Can you work these out from the model? Positions are in its coordinate system, mm. A direction names the side the tool comes from. Give positions to 0.01 mm unless a question says otherwise; leave off trailing zeros. Loops run counter-clockwise (first coordinate to the right, second up) from the corner with the lowest first, then second, coordinate; pieces in that order, holes last. Notation, with made-up numbers: M 81.5,65.25 L 119.5,65.25 A33 cw 119.5,95.25 Z; hole C 50,16 d11. An arc over 180 degrees is marked long. Use CSV: the item, a comma, the result in double quotes.
Autodesk Fusion 360 part; units mm, degrees
sketch "Sketch1" plane through (0, 0, 0) normal (0, 1, 0) x (1, 0, 0)
  line L0 (-6.9154, 10.127) -> (7.6855, 10.127)
  line L1 (7.6855, 10.127) -> (7.6855, -8.5945)
  line L2 (7.6855, -8.5945) -> (-6.9154, -8.5945)
  line L3 (-6.9154, -8.5945) -> (-6.9154, 10.127)
extrude "Extrude1" add sketch "Sketch1" along normal blind 6
sketch "Sketch2" plane through (0, 0, 0) normal (0, -1, 0) x (1, 0, 0)
  line L0 (7.6855, 8.5945) -> (-6.9154, 8.5945)
  line L1 (-6.9154, 8.5945) -> (-6.9154, -10.127)
  line L2 (-6.9154, -10.127) -> (7.6855, -10.127)
  line L3 (7.6855, -10.127) -> (7.6855, 8.5945)
  line L4 (-6.9154, 8.5945) -> (-4.4154, 8.5945)
  line L5 (7.6855, 8.5945) -> (5.1855, 8.5945)
  line L6 (-4.4154, 8.5945) -> (-4.4154, 7.6945)
  line L7 (5.1855, 8.5945) -> (5.1855, 7.6945)
  line L8 (5.1855, 7.6945) -> (5.1855, 3.6245)
  line L9 (-4.4154, 7.6945) -> (5.1855, 7.6945)
  line L10 (5.1855, 7.6945) -> (5.1855, 3.6245)
  line L11 (5.1855, 3.6245) -> (-4.4154, 3.6245)
  line L12 (-4.4154, 3.6245) -> (-4.4154, 7.6945)
  dimension "d3" = 2.5
  dimension "d4" = 2.5
  dimension "d5" = 0.9
  dimension "d6" = 0.9
  dimension "d7" = 4.07
extrude "Extrude2" cut sketch "Sketch2" against normal blind 4.5 contours L8 L9 L10 L11 L12
sketch "Sketch3" plane through (-6.9154, 0, 0) normal (-1, 0, 0) x (0, 0, 1)
  line L0 (-10.127, 0) -> (8.5945, 0)
  line L1 (8.5945, 0) -> (8.5945, 6)
  line L2 (8.5945, 6) -> (-10.127, 6)
  line L3 (-10.127, 6) -> (-10.127, 0)
  line L4 (8.5945, 0) -> (3.6345, 0)
  line L5 (8.5945, 0) -> (7.6945, 0)
  line L6 (7.6945, 0) -> (7.6945, 4.5)
  line L7 (3.6345, 0) -> (3.6245, 4.5)
  dimension "d10" = 4.96
  dimension "d11" = 0.9
  dimension "d12" = 4.5
sketch "Sketch4" plane through (0, 6, 0) normal (0, 1, 0) x (-1, 0, 0)
  line L0 (6.9154, 8.5945) -> (-7.6855, 8.5945)
  line L1 (-7.6855, 8.5945) -> (-7.6855, -10.127)
  line L2 (-7.6855, -10.127) -> (6.9154, -10.127)
  line L3 (6.9154, -10.127) -> (6.9154, 8.5945)
  line L4 (6.9154, 8.5945) -> (4.9154, 8.5945)
  line L5 (-7.6855, 8.5945) -> (-5.6855, 8.5945)
  line L6 (6.9154, -10.127) -> (4.9154, -10.127)
  line L7 (-7.6855, -10.127) -> (-5.6855, -10.127)
  line L8 (4.9154, -10.127) -> (-5.6855, -10.127)
  line L9 (-5.6855, -10.127) -> (-5.6855, 8.5945)
  line L10 (-5.6855, 8.5945) -> (4.9154, 8.5945)
  line L11 (4.9154, 8.5945) -> (4.9154, -10.127)
  dimension "d13" = 2
  dimension "d14" = 2
  dimension "d15" = 2
  dimension "d16" = 2
extrude "Extrude3" cut sketch "Sketch4" against normal up to surface (1.5 mm away) contours L0 L2 L8 L9 L10 L11
sketch "Sketch5" plane through (0, 0, 8.5945) normal (0, 0, 1) x (1, 0, 0)
  line L0 (-4.9154, 4.5) -> (-4.9154, 6)
  line L1 (-4.9154, 6) -> (-6.9154, 6)
  line L2 (-6.9154, 6) -> (-6.9154, 0)
  line L3 (-6.9154, 0) -> (7.6855, 0)
  line L4 (7.6855, 0) -> (7.6855, 6)
  line L5 (7.6855, 6) -> (5.6855, 6)
  line L6 (5.6855, 6) -> (5.6855, 4.5)
  line L7 (5.6855, 4.5) -> (-4.9154, 4.5)
  line L8 (-4.9154, 4.5) -> (-5.9154, 4.5)
  line L9 (5.6855, 4.5) -> (6.6855, 4.5)
  line L10 (-5.9154, 4.5) -> (-5.9154, 5.6)
  line L11 (6.6855, 4.5) -> (6.6855, 5.6)
  line L12 (-4.9154, 4.5) -> (-5.9154, 4.5)
  line L13 (-5.9154, 4.5) -> (-5.9154, 5.6)
  line L14 (-5.9154, 5.6) -> (-4.9154, 5.6)
  line L15 (-4.9154, 5.6) -> (-4.9154, 4.5)
  line L16 (5.6855, 4.5) -> (6.6855, 4.5)
  line L17 (6.6855, 4.5) -> (6.6855, 5.6)
  line L18 (6.6855, 5.6) -> (5.6855, 5.6)
  line L19 (5.6855, 5.6) -> (5.6855, 4.5)
  dimension "d19" = 1
  dimension "d20" = 1
  dimension "d21" = 1.1
  dimension "d22" = 1.1
extrude "Extrude5" cut sketch "Sketch5" against normal up to surface (18.7215 mm away) contours L6 L9 L11 L16 L17 L18 L19
extrude "Extrude4" cut sketch "Sketch5" against normal up to surface (18.7215 mm away) contours L0 L8 L10 L12 L13 L14 L15
sketch "Sketch6" plane through (0, 4.5, 0) normal (0, 1, 0) x (-1, 0, 0)
  line L0 (-5.1855, 3.6245) -> (-5.1855, 7.6945)
  line L1 (-5.1855, 7.6945) -> (4.4154, 7.6945)
  line L2 (4.4154, 7.6945) -> (4.4154, 3.6245)
  line L3 (4.4154, 3.6245) -> (-5.1855, 3.6245)
  line L4 (-6.6855, -10.127) -> (5.9154, -10.127)
  line L5 (5.9154, -10.127) -> (5.9154, 8.5945)
  line L6 (5.9154, 8.5945) -> (-6.6855, 8.5945)
  line L7 (-6.6855, 8.5945) -> (-6.6855, -10.127)
  line L8 (4.4154, 7.6945) -> (-5.1855, 7.6945)
  line L9 (-5.1855, 7.6945) -> (-5.1855, 8.5945)
  line L10 (-5.1855, 8.5945) -> (4.4154, 8.5945)
  line L11 (4.4154, 8.5945) -> (4.4154, 7.6945)
extrude "Extrude6" cut sketch "Sketch6" against normal up to surface (4.5 mm away) contours L1 L6 L8 L9 L10 L11
fillet "Fillet1" radius 0.05 6 edges at (5.6855, 5.6, -0.7662) (6.1855, 5.6, 8.5945) (6.6855, 5.05, 8.5945) (5.9355, 4.5, 8.5945) (5.1855, 4.5, 6.1095) (0.3851, 4.5, 3.6245)
fillet "Fillet2" radius 0.05 13 edges at (-4.4154, 2.225, 3.6245) (-4.4154, 4.4854, 3.6099) (-4.4154, 2.25, 8.5945) (0.3851, 0, 3.6245) (5.1855, 2.225, 3.6245) (5.2001, 4.4854, 3.6099) (5.1855, 0, 6.1095) (-4.4154, 0, 6.1095) (-4.4154, 4.5, 6.0845) (-5.1654, 4.5, 8.5945) (-5.9154, 5.05, 8.5945) (-5.4154, 5.6, 8.5945) (-5.9154, 4.5, -0.7662)
fillet "Fillet3" radius 0.05 4 edges at (6.6855, 5.05, -10.127) (-5.9154, 5.075, -10.127) (-5.9007, 4.5146, -10.127) (0.4101, 4.5, -10.127)
Q1. I want a section at C-C, the plane x = 6. Please give me the cut outline in (y, z), then the cut area to 3 significant figures.
Model answer:
outline,"M 0,-10.13 L 4.45,-10.13 A0.05 ccw 4.5,-10.08 L 4.5,8.54 A0.05 ccw 4.45,8.59 L 0,8.59 Z; M 5.6,-10.13 L 6,-10.13 L 6,8.59 L 5.65,8.59 A0.05 ccw 5.6,8.54 Z"
area,"91.7 mm2"
Q2. I want a section at A-A, the plane y = 5. Please give me the cut outline in (x, z).
Model answer:
outline,"M -6.92,-10.13 L -5.97,-10.13 A0.05 ccw -5.92,-10.08 L -5.92,8.54 A0.05 ccw -5.97,8.59 L -6.92,8.59 Z; M 6.69,-10.08 A0.05 ccw 6.74,-10.13 L 7.69,-10.13 L 7.69,8.59 L 6.74,8.59 A0.05 ccw 6.69,8.54 Z"
Q3. For faces 1 (the flat face through (7.686, 3, -1)), 2 (the flat face through (5.186, 2, 6)), 3 (the flat face through (6, 5.6, -1)), which set-ups out of +Z, -Z, +X, -X, +Y, -Y let a thin tool reach every point of the face, with its end or its side?
Model answer:
face 1,"+Z, -Z, +X, +Y, -Y"
face 2,"+Z, +Y, -Y"
face 3,"+Z, -Z"
Q4. If we mould it in two halves opening along Y, with no side actions, what happens to faces 4 (the flat face through (6.686, 5, -1)), 5 (the flat face through (0, 2, 3.624)), 6 (the flat face through (-5.915, 5, -1)), 7 (the flat face through (7, 6, -1))? For each: released by +Y, released by -Y, zero draft, split by the parting line, or undercut.
Model answer:
face 4,"undercut"
face 5,"zero draft"
face 6,"undercut"
face 7,"released by +Y"
Q5. I'm going to push flat-ended pins straight in: P1, Ø0.5, axis at x = 6, z = -3.5, coming from the -Y side; P2, Ø2, axis at x = 2, y = 1.5, coming from the +Z side. Where does each tip first touch, or does it pass through?
Model answer:
P1,"y = 0"
P2,"z = 3.62"
Q6. I want a section at D-D, the plane x = -2.25. Please give me the cut outline in (y, z), then the cut area to 3 significant figures.
Model answer:
outline,"M 0,-10.13 L 4.45,-10.13 A0.05 ccw 4.5,-10.08 L 4.5,3.57 A0.05 ccw 4.45,3.62 L 0.05,3.62 A0.05 ccw 0,3.57 Z"
area,"61.9 mm2"
Q7. I want a section at B-B, the plane z = 7. Please give me the cut outline in (x, y).
Model answer:
outline,"M -6.92,0 L -4.47,0 A0.05 ccw -4.42,0.05 L -4.42,4.45 A0.05 ccw -4.47,4.5 L -5.87,4.5 A0.05 cw -5.92,4.55 L -5.92,5.6 L -4.92,5.6 L -4.92,6 L -6.92,6 Z; M 5.19,0.05 A0.05 ccw 5.24,0 L 7.69,0 L 7.69,6 L 5.69,6 L 5.69,5.65 A0.05 ccw 5.74,5.6 L 6.69,5.6 L 6.69,4.5 L 5.24,4.5 A0.05 ccw 5.19,4.45 Z"
Q8. Please list where these lines run through material, in increasing order: L1, parallel to X at y = 5.5, z = 2.5; L2, parallel to Y at x = -5, z = -3.5; L3, parallel to X at y = 4.25, z = 6.5. Write a range as from..to.
Model answer:
L1,"-6.92..-5.92, 6.69..7.69"
L2,"0..4.5, 5.6..6"
L3,"-6.92..-4.42, 5.19..7.69"
